Read the model definition and answer for the solid it produces. Units are mm, in the model's axes. Face numbers are marked on the shaded views. Round coordinates to 2 decimals unless told otherwise and drop trailing zeros. Loops run counter-clockwise (first coordinate to the right, second up) from the corner with the lowest first, then second, coordinate; pieces in that order, holes last. Notation, with made-up numbers: M 66.5,75 L 109.5,75 A24 ccw 109.5,102 Z; hole C 22,65 d5. An arc over 180 degrees is marked long. Write each question's results on one line, items separated by ' | '.
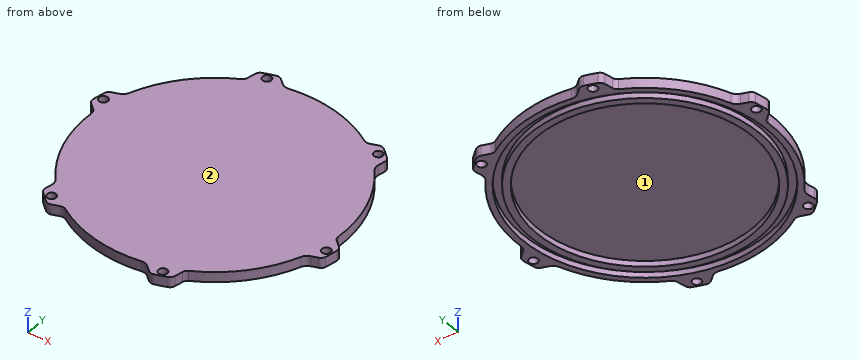
from build123d import *

# Parameters (mm, degrees)
SKETCH2_R             = 39.4
BOSS_EXTRUDE1_DEPTH   = 2
SKETCH2_R_2           = 1.5
SKETCH2_R_3           = 42
BOSS_EXTRUDE1_2_DEPTH = 2
SKETCH3_R             = 1.5
BOSS_EXTRUDE2_DEPTH   = 1.5
SKETCH4_R             = 37
CUT_EXTRUDE1_DEPTH    = 2


with BuildPart() as part:
    # Sketch2 → Boss-Extrude1 (new body)
    with BuildSketch(Plane.XY):
        Circle(SKETCH2_R)
    extrude(amount=BOSS_EXTRUDE1_DEPTH)



with BuildPart() as body_2:
    # Sketch2 → Boss-Extrude1 2 (new body)
    with BuildSketch(Plane.XY):
        with BuildLine():
            Line((-45.018479974, 13.897886094), (-42.708823016, 14.636743864))
            ThreePointArc((-42.708823016, 14.636743864), (-41.579055756, 15.298025015), (-40.838449582, 16.377455105))
            ThreePointArc((-40.838449582, 16.377455105), (-32.228172293, 29.955715826), (-19.314601011, 39.534114228))
            ThreePointArc((-19.314601011, 39.534114228), (-18.626580504, 40.087021781), (-18.243561026, 40.882241915))
            Line((-18.243561026, 40.882241915), (-17.592978184, 43.707000534))
            ThreePointArc((-17.592978184, 43.707000534), (-17.140898521, 44.584509163), (-16.324175781, 45.138910987))
            ThreePointArc((-16.324175781, 45.138910987), (-14.341791733, 45.80734668), (-12.332164177, 46.388767247))
            ThreePointArc((-12.332164177, 46.388767247), (-11.345102668, 46.399111036), (-10.473317571, 45.936090345))
            Line((-10.473317571, 45.936090345), (-8.678619493, 44.30529763))
            ThreePointArc((-8.678619493, 44.30529763), (-7.541049587, 43.657531057), (-6.235932621, 43.555862342))
            ThreePointArc((-6.235932621, 43.555862342), (9.828324748, 42.888273836), (24.580246732, 36.493992253))
            ThreePointArc((24.580246732, 36.493992253), (25.403088973, 36.174602792), (26.283279549, 36.240508262))
            Line((26.283279549, 36.240508262), (29.054883694, 37.089466303))
            ThreePointArc((29.054883694, 37.089466303), (30.04086829, 37.136708144), (30.929355724, 36.706606415))
            ThreePointArc((30.929355724, 36.706606415), (32.499430039, 35.324029316), (34.007768798, 33.874351084))
            ThreePointArc((34.007768798, 33.874351084), (34.510257536, 33.024702637), (34.545162404, 32.03820425))
            Line((34.545162404, 32.03820425), (34.030203523, 29.668553765))
            ThreePointArc((34.030203523, 29.668553765), (34.038006169, 28.359506042), (34.602516962, 27.178407237))
            ThreePointArc((34.602516962, 27.178407237), (42.05649704, 12.93255801), (43.894847743, -3.040121975))
            ThreePointArc((43.894847743, -3.040121975), (44.029669477, -3.912418989), (44.526840575, -4.641733653))
            Line((44.526840575, -4.641733653), (46.647861878, -6.617534232))
            ThreePointArc((46.647861878, -6.617534232), (47.181766811, -7.447801019), (47.253531504, -8.432304572))
            ThreePointArc((47.253531504, -8.432304572), (46.841221772, -10.483317364), (46.339932975, -12.514416163))
            ThreePointArc((46.339932975, -12.514416163), (45.855360204, -13.374408399), (45.018479974, -13.897886094))
            Line((45.018479974, -13.897886094), (42.708823016, -14.636743864))
            ThreePointArc((42.708823016, -14.636743864), (41.579055756, -15.298025015), (40.838449582, -16.377455105))
            ThreePointArc((40.838449582, -16.377455105), (32.228172293, -29.955715826), (19.314601011, -39.534114228))
            ThreePointArc((19.314601011, -39.534114228), (18.626580504, -40.087021781), (18.243561026, -40.882241915))
            Line((18.243561026, -40.882241915), (17.592978184, -43.707000534))
            ThreePointArc((17.592978184, -43.707000534), (17.140898521, -44.584509163), (16.324175781, -45.138910987))
            ThreePointArc((16.324175781, -45.138910987), (14.341791733, -45.80734668), (12.332164177, -46.388767247))
            ThreePointArc((12.332164177, -46.388767247), (11.345102668, -46.399111036), (10.473317571, -45.936090345))
            Line((10.473317571, -45.936090345), (8.678619493, -44.30529763))
            ThreePointArc((8.678619493, -44.30529763), (7.541049587, -43.657531057), (6.235932621, -43.555862342))
            ThreePointArc((6.235932621, -43.555862342), (-9.828324748, -42.888273836), (-24.580246732, -36.493992253))
            ThreePointArc((-24.580246732, -36.493992253), (-25.403088973, -36.174602792), (-26.283279549, -36.240508262))
            Line((-26.283279549, -36.240508262), (-29.054883694, -37.089466303))
            ThreePointArc((-29.054883694, -37.089466303), (-30.04086829, -37.136708144), (-30.929355724, -36.706606415))
            ThreePointArc((-30.929355724, -36.706606415), (-32.499430039, -35.324029316), (-34.007768798, -33.874351084))
            ThreePointArc((-34.007768798, -33.874351084), (-34.510257536, -33.024702637), (-34.545162404, -32.03820425))
            Line((-34.545162404, -32.03820425), (-34.030203523, -29.668553765))
            ThreePointArc((-34.030203523, -29.668553765), (-34.038006169, -28.359506042), (-34.602516962, -27.178407237))
            ThreePointArc((-34.602516962, -27.178407237), (-42.05649704, -12.93255801), (-43.894847743, 3.040121975))
            ThreePointArc((-43.894847743, 3.040121975), (-44.029669477, 3.912418989), (-44.526840575, 4.641733653))
            Line((-44.526840575, 4.641733653), (-46.647861878, 6.617534232))
            ThreePointArc((-46.647861878, 6.617534232), (-47.181766811, 7.447801019), (-47.253531504, 8.432304572))
            ThreePointArc((-47.253531504, 8.432304572), (-46.841221772, 10.483317364), (-46.339932975, 12.514416163))
            ThreePointArc((-46.339932975, 12.514416163), (-45.855360204, 13.374408399), (-45.018479974, 13.897886094))
        make_face()
        with Locations((-13.744217077, 43.898707235)):
            Circle(SKETCH2_R_2, mode=Mode.SUBTRACT)
        with Locations((-44.889504198, 10.046512474)):
            Circle(SKETCH2_R_2, mode=Mode.SUBTRACT)
        with Locations((31.145287121, 33.852194762)):
            Circle(SKETCH2_R_2, mode=Mode.SUBTRACT)
        with Locations((44.889504198, -10.046512474)):
            Circle(SKETCH2_R_2, mode=Mode.SUBTRACT)
        with Locations((13.744217077, -43.898707235)):
            Circle(SKETCH2_R_2, mode=Mode.SUBTRACT)
        with Locations((-31.145287121, -33.852194762)):
            Circle(SKETCH2_R_2, mode=Mode.SUBTRACT)
        Circle(SKETCH2_R_3, mode=Mode.SUBTRACT)
    extrude(amount=BOSS_EXTRUDE1_2_DEPTH)


with BuildPart() as part_1:
    add(part.part)

    add(body_2.part)  # Boss-Extrude2 merges body 2
    # Sketch3 → Boss-Extrude2 (add)
    with BuildSketch(Plane.XY.offset(2)):
        with BuildLine():
            Line((8.678619493, -44.30529763), (10.473317571, -45.936090345))
            ThreePointArc((10.473317571, -45.936090345), (11.345102668, -46.399111036), (12.332164177, -46.388767247))
            ThreePointArc((12.332164177, -46.388767247), (14.341791733, -45.80734668), (16.324175781, -45.138910987))
            ThreePointArc((16.324175781, -45.138910987), (17.140898521, -44.584509163), (17.592978184, -43.707000534))
            Line((17.592978184, -43.707000534), (18.243561026, -40.882241915))
            ThreePointArc((18.243561026, -40.882241915), (18.626580504, -40.087021781), (19.314601011, -39.534114228))
            ThreePointArc((19.314601011, -39.534114228), (32.228172293, -29.955715826), (40.838449582, -16.377455105))
            ThreePointArc((40.838449582, -16.377455105), (41.579055756, -15.298025015), (42.708823016, -14.636743864))
            Line((42.708823016, -14.636743864), (45.018479974, -13.897886094))
            ThreePointArc((45.018479974, -13.897886094), (45.855360204, -13.374408399), (46.339932975, -12.514416163))
            ThreePointArc((46.339932975, -12.514416163), (46.841221772, -10.483317364), (47.253531504, -8.432304572))
            ThreePointArc((47.253531504, -8.432304572), (47.181766811, -7.447801019), (46.647861878, -6.617534232))
            Line((46.647861878, -6.617534232), (44.526840575, -4.641733653))
            ThreePointArc((44.526840575, -4.641733653), (44.029669477, -3.912418989), (43.894847743, -3.040121975))
            ThreePointArc((43.894847743, -3.040121975), (42.05649704, 12.93255801), (34.602516962, 27.178407237))
            ThreePointArc((34.602516962, 27.178407237), (34.038006169, 28.359506042), (34.030203523, 29.668553765))
            Line((34.030203523, 29.668553765), (34.545162404, 32.03820425))
            ThreePointArc((34.545162404, 32.03820425), (34.510257536, 33.024702637), (34.007768798, 33.874351084))
            ThreePointArc((34.007768798, 33.874351084), (32.499430039, 35.324029316), (30.929355724, 36.706606415))
            ThreePointArc((30.929355724, 36.706606415), (30.04086829, 37.136708144), (29.054883694, 37.089466303))
            Line((29.054883694, 37.089466303), (26.283279549, 36.240508262))
            ThreePointArc((26.283279549, 36.240508262), (25.403088973, 36.174602792), (24.580246732, 36.493992253))
            ThreePointArc((24.580246732, 36.493992253), (9.828324748, 42.888273836), (-6.235932621, 43.555862342))
            ThreePointArc((-6.235932621, 43.555862342), (-7.541049587, 43.657531057), (-8.678619493, 44.30529763))
            Line((-8.678619493, 44.30529763), (-10.473317571, 45.936090345))
            ThreePointArc((-10.473317571, 45.936090345), (-11.345102668, 46.399111036), (-12.332164177, 46.388767247))
            ThreePointArc((-12.332164177, 46.388767247), (-14.341791733, 45.80734668), (-16.324175781, 45.138910987))
            ThreePointArc((-16.324175781, 45.138910987), (-17.140898521, 44.584509163), (-17.592978184, 43.707000534))
            Line((-17.592978184, 43.707000534), (-18.243561026, 40.882241915))
            ThreePointArc((-18.243561026, 40.882241915), (-18.626580504, 40.087021781), (-19.314601011, 39.534114228))
            ThreePointArc((-19.314601011, 39.534114228), (-32.228172293, 29.955715826), (-40.838449582, 16.377455105))
            ThreePointArc((-40.838449582, 16.377455105), (-41.579055756, 15.298025015), (-42.708823016, 14.636743864))
            Line((-42.708823016, 14.636743864), (-45.018479974, 13.897886094))
            ThreePointArc((-45.018479974, 13.897886094), (-45.855360204, 13.374408399), (-46.339932975, 12.514416163))
            ThreePointArc((-46.339932975, 12.514416163), (-46.841221772, 10.483317364), (-47.253531504, 8.432304572))
            ThreePointArc((-47.253531504, 8.432304572), (-47.181766811, 7.447801019), (-46.647861878, 6.617534232))
            Line((-46.647861878, 6.617534232), (-44.526840575, 4.641733653))
            ThreePointArc((-44.526840575, 4.641733653), (-44.029669477, 3.912418989), (-43.894847743, 3.040121975))
            ThreePointArc((-43.894847743, 3.040121975), (-42.05649704, -12.93255801), (-34.602516962, -27.178407237))
            ThreePointArc((-34.602516962, -27.178407237), (-34.038006169, -28.359506042), (-34.030203523, -29.668553765))
            Line((-34.030203523, -29.668553765), (-34.545162404, -32.03820425))
            ThreePointArc((-34.545162404, -32.03820425), (-34.510257536, -33.024702637), (-34.007768798, -33.874351084))
            ThreePointArc((-34.007768798, -33.874351084), (-32.499430039, -35.324029316), (-30.929355724, -36.706606415))
            ThreePointArc((-30.929355724, -36.706606415), (-30.04086829, -37.136708144), (-29.054883694, -37.089466303))
            Line((-29.054883694, -37.089466303), (-26.283279549, -36.240508262))
            ThreePointArc((-26.283279549, -36.240508262), (-25.403088973, -36.174602792), (-24.580246732, -36.493992253))
            ThreePointArc((-24.580246732, -36.493992253), (-9.828324748, -42.888273836), (6.235932621, -43.555862342))
            ThreePointArc((6.235932621, -43.555862342), (7.541049587, -43.657531057), (8.678619493, -44.30529763))
        make_face()
        with Locations((-13.744217077, 43.898707235)):
            Circle(SKETCH3_R, mode=Mode.SUBTRACT)
        with Locations((31.145287121, 33.852194762)):
            Circle(SKETCH3_R, mode=Mode.SUBTRACT)
        with Locations((-44.889504198, 10.046512474)):
            Circle(SKETCH3_R, mode=Mode.SUBTRACT)
        with Locations((-31.145287121, -33.852194762)):
            Circle(SKETCH3_R, mode=Mode.SUBTRACT)
        with Locations((13.744217077, -43.898707235)):
            Circle(SKETCH3_R, mode=Mode.SUBTRACT)
        with Locations((44.889504198, -10.046512474)):
            Circle(SKETCH3_R, mode=Mode.SUBTRACT)
    extrude(amount=BOSS_EXTRUDE2_DEPTH)

    # Sketch4 → Cut-Extrude1 (cut)
    with BuildSketch(Plane(origin=(0, 0, 0), x_dir=(-1, 0, 0), z_dir=(0, 0, -1))):
        Circle(SKETCH4_R)
    extrude(amount=-CUT_EXTRUDE1_DEPTH, mode=Mode.SUBTRACT)


solid = part_1.part
Item 1: The mould has two halves that part along X. Classify the marked faces 1 and 2: pulls with the +X half, pulls with the -X half, needs draft (parallel to the pull), parting line crosses it, or undercut.
Outcome:
face 1: undercut | face 2: needs draft
Item 2: Flat-ended cylindrical pins translate along their axes: pin 1 (3.5 mm diameter, centred on x = -13.74, y = 43.9, fed in from -Z); pin 2 (25 mm diameter, centred on x = -5.5, y = 17.5, fed in from -Z); pin 3 (1.5 mm diameter, centred on x = -24.5, z = 0.5, fed in from -Y); pin 4 (1 mm diameter, centred on y = 25.5, z = 1, fed in from +X). Find the tip coordinate at first contact, or state that the pin passes through.
Outcome:
pin 1: stops at z = 0 | pin 2: stops at z = 2 | pin 3: stops at y = -37.04 | pin 4: stops at x = 36.21
Item 3: The part is cut by section A-A (x = 0). Determine the outline of the cut face in (y, z), plus the area to 3 significant figures.
Outcome:
outline: M -44,0 L -42,0 L -42,2 L -39.4,2 L -39.4,0 L -37,0 L -37,2 L 37,2 L 37,0 L 39.4,0 L 39.4,2 L 42,2 L 42,0 L 44,0 L 44,3.5 L -44,3.5 Z | area: 150 mm2
Item 4: The part is cut by section C-C (z = 1.15). State how many separate pieces and enclosed holes the cut face has, plus the area to 3 significant figures.
Outcome:
separate pieces: 2 | enclosed holes: 8 | area: 1,290 mm2
Item 5: Straight lines are drawn through the part: line 1 (X direction, y = -1, z = 0.85); line 2 (X direction, y = -22, z = 1.35); line 3 (Y direction, x = -10, z = 0.4). For each, find the intervals that lie inside material, in ascending order.
Outcome:
line 1: x = -43.99 to -41.99, -39.39 to -36.99, 36.99 to 39.39, 41.99 to 43.99 | line 2: x = -38.11 to -35.78, -32.69 to -29.75, 29.75 to 32.69, 35.78 to 38.11 | line 3: y = -42.85 to -40.79, -38.11 to -35.62, 35.62 to 38.11, 40.79 to 45.51
